Verification items for this drawing (mm, ordinates from the low corner). Give positions to 0.01 mm unless a question says otherwise; leave off trailing zeros. Loops run counter-clockwise (first coordinate to the right, second up) from the corner with the lowest first, then second, coordinate; pieces in that order, holes last. Notation, with made-up numbers: (-39.75, 27) -> (4.25, 27) arc R17 cw to (4.25, 60) -> close; hole circle Ø4 at (-3.75, -5.5). An arc over 180 degrees is marked (long way). Use one line per item in the form item = value. Start each with the question number.
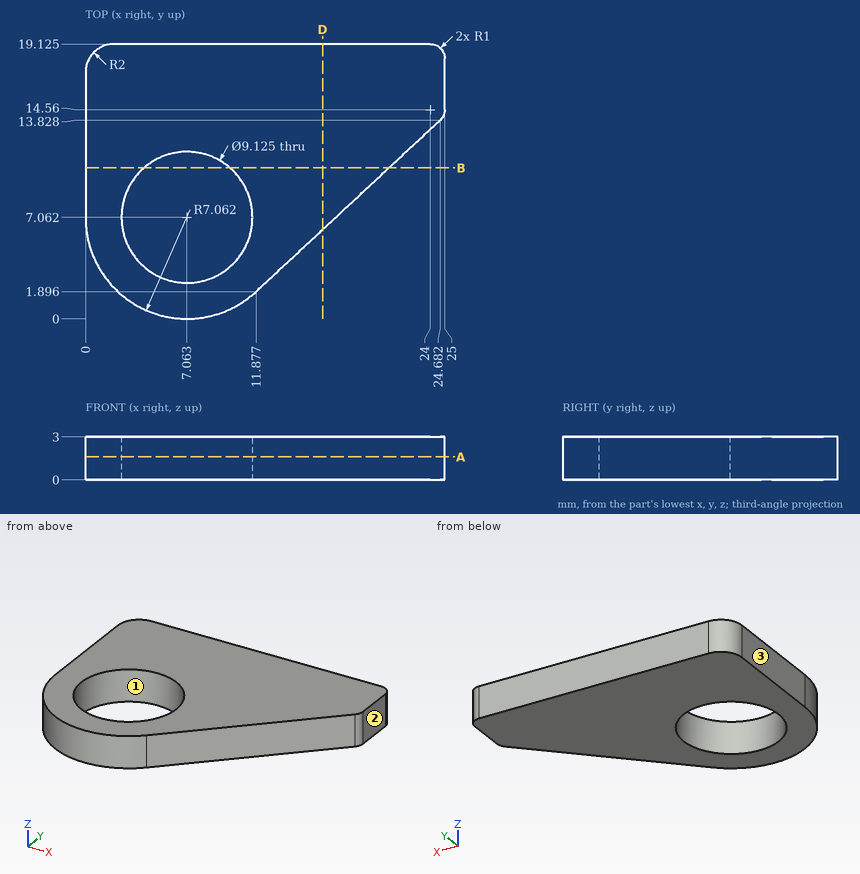
Item 1: Gauge pin test, flat end, axial feed: pin 1 Ø1 at (x, z) = (22, 2.5) entering from -Y (1 decimal). Record the tip position at first contact, or that the pin passes through.
Item 2: Sectioned sample at D-D, the plane x = 16.5. Enter the section's corners in (y, z) (1 decimal).
Item 3: Sectioned sample at B-B, the plane y = 10.5. Enter the section's corners in (x, z).
Item 4: Sectioned sample at A-A, the plane z = 1.6. Enter the section's corners in (x, y) (1 decimal), and give its area (3 significant figures).
Item 5: Material ranges on line 1 (Y direction, x = 3.25, z = 2.5) (1 decimal); line 2 (X direction, y = 10.5, z = 0.1) (1 decimal); line 3 (X direction, y = 4, z = 0.8) (1 decimal), recorded low to high.
Item 6: Draft check along X on the marked faces 1, 2 and 3. Enter one of: +X half, -X half, draft (parallel to the pull), parting line (faces both ways), or undercut.
Outcome:
q1.pin_1 = 10.9
q2.outline = (6.2, 0) -> (19.1, 0) -> (19.1, 3) -> (6.2, 3) -> close
q3.outline = (0, 0) -> (4.06, 0) -> (4.06, 3) -> (0, 3) -> close; (10.06, 0) -> (21.11, 0) -> (21.11, 3) -> (10.06, 3) -> close
q4.outline = (0, 7.1) arc R7.1 ccw to (11.9, 1.9) -> (24.7, 13.8) arc R1 ccw to (25, 14.6) -> (25, 18.1) arc R1 ccw to (24, 19.1) -> (2, 19.1) arc R2 ccw to (0, 17.1) -> close; hole circle Ø9.1 at (7.1, 7.1)
q4.area = 293 mm^2
q5.line_1 = 1.1 to 4.6, 9.6 to 19.1
q5.line_2 = 0 to 4.1, 10.1 to 21.1
q5.line_3 = 0.7 to 3.7, 10.4 to 14.1
q6.face_1 = undercut
q6.face_2 = +X half
q6.face_3 = -X half
